```python
from build123d import *

# Parameters (mm, degrees)
BOSS_EXTRUDE2_DEPTH = 2.54
SKETCH5_W           = 0.635
SKETCH5_H           = 0.635
SKETCH6_W           = 0.635
SKETCH6_H           = 0.635
CHAMFER1_SIZE       = 0.1905


with BuildPart() as part:
    # Sketch1 → Boss-Extrude2 (new body)
    with BuildSketch(Plane(origin=(0, 0, 0), x_dir=(1, 0, 0), z_dir=(0, 1, 0))):
        Polygon((-2.413, -0.762), (-1.651, -1.27), (1.651, -1.27), (2.413, -0.762), (2.413, 0.762), (1.651, 1.27), (-1.651, 1.27), (-2.413, 0.762), align=None)
    extrude(amount=BOSS_EXTRUDE2_DEPTH)

    # Sweep5: sweep along a path in Sketch2
    with BuildLine(Plane.XY) as sweep5_path:
        Line((-1.27, 7.62), (-1.27, 2.54))
        Line((-1.27, 2.54), (-1.27, -0.889))
        ThreePointArc((-1.27, -0.889), (-1.455987194, -1.338012806), (-1.905, -1.524))
        Line((-1.905, -1.524), (-4.953, -1.524))
    # Sketch5 → Sweep5 (sweep)
    with BuildSketch(Plane(origin=(0, 7.62, 0), x_dir=(1, 0, 0), z_dir=(0, 1, 0))):
        with Locations((-1.27, 0)):
            Rectangle(SKETCH5_W, SKETCH5_H)
    sweep(path=sweep5_path.line)

    # Sweep6: sweep along a path in Sketch7
    with BuildLine(Plane.XY) as sweep6_path:
        Line((-4.953, -4.064), (0.635, -4.064))
        ThreePointArc((0.635, -4.064), (1.084012806, -3.878012806), (1.27, -3.429))
        Line((1.27, -3.429), (1.27, 2.54))
        Line((1.27, 2.54), (1.27, 7.62))
    # Sketch6 → Sweep6 (sweep)
    with BuildSketch(Plane(origin=(0, 7.62, 0), x_dir=(1, 0, 0), z_dir=(0, 1, 0))):
        with Locations((1.27, 0)):
            Rectangle(SKETCH6_W, SKETCH6_H)
    sweep(path=sweep6_path.line)

    # Chamfer1
    chamfer1_edges = [part.edges().sort_by_distance(p)[0] for p in [
        (-4.953, -1.524, -0.3175),
        (-4.953, -1.8415, 0),
        (-4.953, -1.524, 0.3175),
        (-4.953, -1.2065, 0),
        (-1.27, 7.62, -0.3175),
        (-0.9525, 7.62, 0),
        (-1.27, 7.62, 0.3175),
        (-1.5875, 7.62, 0),
        (1.5875, 7.62, 0),
        (1.27, 7.62, -0.3175),
        (0.9525, 7.62, 0),
        (1.27, 7.62, 0.3175),
        (-4.953, -4.3815, 0),
        (-4.953, -4.064, -0.3175),
        (-4.953, -3.7465, 0),
        (-4.953, -4.064, 0.3175),
    ]]
    chamfer(chamfer1_edges, length=CHAMFER1_SIZE)

    # Mirror1: part across plane


with BuildPart() as part_1:
    add(part.part)
    add(part.part.mirror(Plane(origin=(-1.651, 2.54, -1.27), x_dir=(1, 0, 0), z_dir=(0, 0, 1))))


solid = part_1.part
```
Model file for the job. Use its own axes, mm. A direction names the side the tool comes from. Coordinates: 2 decimals unless noted, no trailing zeros. Order: outer loops, then holes, each group sorted by start corner. A loop starts at its lowest first (then second) coordinate and runs counter-clockwise, first axis right, second up. Notation, with made-up numbers: (16, 6.5) -> (21, 6.5) arc R20 cw to (21, 32.5) -> close; hole circle Ø5 at (-26, -31.75). An arc over 180 degrees is marked (long way). Answer as a JSON object with one key per item and string values. Group by question number.
1) Cut at C-C, the plane x = -2.25. Write the cut outline in (y, z).
2) Drill centre lines: L1, parallel to Y at x = -0.5, z = -0.25; L2, parallel to Z at x = 1.5, y = 3.5; L3, parallel to Y at x = -3.25, z = -2.55. Where is each one in solid material? Low to high.
3) Cut at B-B, the plane x = -0.5. Write the cut outline in (y, z), then the cut area to 3 significant figures.
4) Cut at A-A, the plane y = -0.25. Write the cut outline in (x, z), then the cut area to 3 significant figures.
5) Flat gauge pins, fed straight in: pin 1 (1.5 mm diameter, centred on x = -3, y = -1, fed in from -Z); pin 2 (0.5 mm diameter, centred on y = -2, z = 0, fed in from -X); pin 3 (0.5 mm diameter, centred on x = -1.5, y = 5, fed in from +Z). Where does each tip first touch, or does it go through?
6) Cut at D-D, the plane z = -3.05. Write the cut outline in (x, y), then the cut area to 3 significant figures.
7) Pull direction X, two halves, no side cores. Call faces 5 (the face through (2.413, 1, 0)), 6 (the face through (-1, -4, -2.858)), 7 (the face through (-1.224, -1.555, -2.536)): +X half, -X half, draft (parallel to the pull), parting line (faces both ways), or undercut.
8) Which spindle directions (+Z, -Z, +X, -X, +Y, -Y) get a long thin tool onto all of the face, cutting with end or side? Do faces 1 (the face through (0, -4, -2.222)), 2 (the face through (-2.5, -1.5, 0.318)), 3 (the face through (-2.5, -1.5, -2.858)), 4 (the face through (-2.413, 1, -3)). Say none if no direction does.
Check values:
{
 "1": {"outline": "(-4.38, -2.86) -> (-3.75, -2.86) -> (-3.75, -2.22) -> (-4.38, -2.22) -> close; (-4.38, -0.32) -> (-3.75, -0.32) -> (-3.75, 0.32) -> (-4.38, 0.32) -> close; (-1.84, -2.86) -> (-1.21, -2.86) -> (-1.21, -2.22) -> (-1.84, -2.22) -> close; (-1.84, -0.32) -> (-1.21, -0.32) -> (-1.21, 0.32) -> (-1.84, 0.32) -> close; (0, -3.41) -> (2.54, -3.41) -> (2.54, -1.67) -> (0, -1.67) -> close; (0, -0.87) -> (2.54, -0.87) -> (2.54, 0.87) -> (0, 0.87) -> close"},
 "2": {"L1": "y = -4.38 to -3.75, 0 to 2.54", "L2": "z = -2.86 to -2.22, -0.32 to 0.32", "L3": "y = -4.38 to -3.75, -1.84 to -1.21"},
 "3": {"outline": "(-4.38, -2.86) -> (-3.75, -2.86) -> (-3.75, -2.22) -> (-4.38, -2.22) -> close; (-4.38, -0.32) -> (-3.75, -0.32) -> (-3.75, 0.32) -> (-4.38, 0.32) -> close; (0, -3.81) -> (2.54, -3.81) -> (2.54, 1.27) -> (0, 1.27) -> close", "area": "13.7 mm²"},
 "4": {"outline": "(-1.59, -2.86) -> (-0.95, -2.86) -> (-0.95, -2.22) -> (-1.59, -2.22) -> close; (-1.59, -0.32) -> (-0.95, -0.32) -> (-0.95, 0.32) -> (-1.59, 0.32) -> close; (0.95, -2.86) -> (1.59, -2.86) -> (1.59, -2.22) -> (0.95, -2.22) -> close; (0.95, -0.32) -> (1.59, -0.32) -> (1.59, 0.32) -> (0.95, 0.32) -> close", "area": "1.61 mm²"},
 "5": {"pin 1": "stops at z = -2.86", "pin 2": "stops at x = -4.85", "pin 3": "stops at z = 0.32"},
 "6": {"outline": "(-2.41, 0) -> (2.41, 0) -> (2.41, 2.54) -> (-2.41, 2.54) -> close", "area": "12.3 mm²"},
 "7": {"face 5": "+X half", "face 6": "draft", "face 7": "undercut"},
 "8": {"face 1": "+X, -X, -Y", "face 2": "+Z, +X, -X, -Y", "face 3": "-Z, +X, -X, -Y", "face 4": "+Z, -Z, -X, +Y"}
}
